Source: CAD feature listing. Evaluate the final solid. Frame: model axes, mm. Give positions to 0.01 mm unless a question says otherwise; leave off trailing zeros. Loops run counter-clockwise (first coordinate to the right, second up) from the corner with the lowest first, then second, coordinate; pieces in that order, holes last. Notation, with made-up numbers: M 23,17 L 43,17 A25 cw 43,30 Z; hole C 37.25,-27.5 d6. An arc over 180 degrees is marked long. Write item = value, one per line.
from build123d import *

# Parameters (mm, degrees)
F2_DEPTH = 12.7


with BuildPart() as f2:
    # F0 (on Front) → F2 (new body)
    with BuildSketch(Plane.XZ):
        with BuildLine():
            ThreePointArc((-9.450293, 115.490625), (-0.596483, 104.793695), (9.525, 114.3))
            ThreePointArc((9.525, 114.3), (9.506305, 114.896483), (9.450293, 115.490625))
            ThreePointArc((9.450293, 115.490625), (0, 123.825), (-9.450293, 115.490625))
        make_face()
        with BuildLine():
            ThreePointArc((9.450293, 115.490625), (9.506305, 114.896483), (9.525, 114.3))
            ThreePointArc((9.525, 114.3), (-0.596483, 104.793695), (-9.450293, 115.490625))
            Line((-9.450293, 115.490625), (-15.750488, 65.484375))
            ThreePointArc((-15.750488, 65.484375), (0, 79.375), (15.750488, 65.484375))
            Line((15.750488, 65.484375), (9.450293, 115.490625))
        make_face()
        with BuildLine():
            ThreePointArc((15.875, 63.5), (15.843841, 64.494139), (15.750488, 65.484375))
            ThreePointArc((15.750488, 65.484375), (0, 79.375), (-15.750488, 65.484375))
            ThreePointArc((-15.750488, 65.484375), (-15.874547, 63.619893), (-15.778664, 61.75375))
            ThreePointArc((-15.778664, 61.75375), (0.630191, 47.637513), (15.867467, 63.011))
            ThreePointArc((15.867467, 63.011), (15.873117, 63.255471), (15.875, 63.5))
        make_face()
        with BuildLine():
            ThreePointArc((15.867467, 63.011), (0.630191, 47.637513), (-15.778664, 61.75375))
            Line((-15.778664, 61.75375), (-8.836052, -0.9779))
            ThreePointArc((-8.836052, -0.9779), (-0.489693, 8.876503), (8.89, 0))
            ThreePointArc((8.89, 0), (6.353174, -6.218463), (0.1905, -8.887959))
            Line((0.1905, -8.887959), (44.620089, -7.935677))
            ThreePointArc((44.620089, -7.935677), (36.545983, 0.728304), (46.067357, 7.770976))
            Line((46.067357, 7.770976), (18.542212, 13.499725))
            ThreePointArc((18.542212, 13.499725), (15.587302, 15.328925), (14.499731, 18.62963))
            Line((14.499731, 18.62963), (15.867467, 63.011))
        make_face()
        with BuildLine():
            ThreePointArc((8.89, 0), (-0.489693, 8.876503), (-8.836052, -0.9779))
            ThreePointArc((-8.836052, -0.9779), (-5.859066, -6.686064), (0.1905, -8.887959))
            ThreePointArc((0.1905, -8.887959), (6.353174, -6.218463), (8.89, 0))
        make_face()
        with BuildLine():
            ThreePointArc((46.067357, 7.770976), (36.545983, 0.728304), (44.620089, -7.935677))
            ThreePointArc((44.620089, -7.935677), (50.122477, -5.552199), (52.3875, 0))
            ThreePointArc((52.3875, 0), (50.60799, 5.0083), (46.067357, 7.770976))
        make_face()
    extrude(amount=F2_DEPTH)


solid = f2.part
1. First-contact query: pin 1 Ø4 at (x, y) = (7, -6.5) entering from -Z; pin 2 Ø1 at (x, y) = (30, -11.5) entering from +Z; pin 3 Ø6 at (y, z) = (-8, 53) entering from -X. Flat tips, straight axial feed; report the tip coordinate or a pass-through.
Derived:
pin_1 = -8.78
pin_2 = 11.22
pin_3 = -15.14
2. Cut plane B-B, the plane x = 29. Return the cut outline in (y, z).
Derived:
outline = M -12.7,-8.27 L 0,-8.27 L 0,11.32 L -12.7,11.32 Z
3. Cut plane C-C, the plane z = 46. Return the cut outline in (x, y).
Derived:
outline = M -14.04,-12.7 L 15.34,-12.7 L 15.34,0 L -14.04,0 Z
4. Pull-direction query (Z, two-part tool) for faces 1 (the cylindrical face through (15.62, -6.26, 15.29)), 2 (the cylindrical face through (-5.928, -6.261, -6.625)), 3 (the cylindrical face through (0.193, -6.261, 123.823)); classes: +Z half, -Z half, draft (parallel to the pull), parting line (faces both ways), or undercut.
Derived:
face_1 = undercut
face_2 = -Z half
face_3 = +Z half
5. Material intervals for probe 1 along X at (y, z) = (-4.5, 66.5); probe 2 along Z at (x, y) = (5, -7.75); probe 3 along Z at (x, y) = (18.5, -4.75), sorted ascending. Write a range as from..to.
Derived:
probe_1 = -15.62..15.62
probe_2 = -8.78..122.41
probe_3 = -8.5..13.51
